Can you work these out from the model? Positions are in its coordinate system, mm. Give positions to 0.01 mm unless a question says otherwise; leave off trailing zeros. Order: outer loops, then holes, each group sorted by start corner. A loop starts at its lowest first (then second) coordinate and runs counter-clockwise, first axis right, second up. Notation, with made-up numbers: (38.25, 48) - (57.25, 48) arc R13 ccw to (57.25, 67) - close; hole circle Ø9 at (78.25, 9.25). An arc over 180 degrees is marked (long way). One line per question, with ' | ' between items.
```python
from build123d import *

# Parameters (mm, degrees)
BOSS_EXTRUDE1_DEPTH      = 3.175
BOSS_EXTRUDE1_DEPTH_BACK = 3.175
CUT_EXTRUDE3_DEPTH       = 206.528461822
CUT_EXTRUDE5_DEPTH       = 206.528461822
CUT_EXTRUDE6_DEPTH       = 6.35
SKETCH8_W                = 3.175
SKETCH8_H                = 3.175
CUT_EXTRUDE7_DEPTH       = 6.35


with BuildPart() as part:
    # Sketch1 → Boss-Extrude1 (new, two sides: drawn at the far end of the back side and taken through both)
    with BuildSketch(Plane.XY.offset(-BOSS_EXTRUDE1_DEPTH_BACK)):
        with BuildLine():
            Line((-95.480291898, -80.706386575), (-95.480291898, -131.085242165))
            Line((-95.480291898, -131.085242165), (-95.480291898, -132.672742165))
            Line((-95.480291898, -132.672742165), (-120.480291898, -132.672742165))
            Line((-120.480291898, -132.672742165), (-120.480291898, -131.085242165))
            Line((-120.480291898, -131.085242165), (-120.480291898, -64.018285781))
            ThreePointArc((-120.480291898, -64.018285781), (-115.755703828, -49.392703021), (-103.367678212, -40.295108567))
            Line((-103.367678212, -40.295108567), (119.519708102, 33.809591006))
            Line((119.519708102, 33.809591006), (119.519708102, 8.809591006))
            Line((119.519708102, 8.809591006), (-78.367678212, -56.983209361))
            ThreePointArc((-78.367678212, -56.983209361), (-90.755703828, -66.080803815), (-95.480291898, -80.706386575))
        make_face()
    extrude(amount=BOSS_EXTRUDE1_DEPTH + BOSS_EXTRUDE1_DEPTH_BACK)

    # Sketch2 → Cut-Extrude3 (cut, through all)
    with BuildSketch(Plane.XZ.offset(132.672742165)):
        Polygon((-120.480291898, 0), (-120.480291898, 3.175), (-118.647204793, 3.175), align=None)
    cut_extrude3 = extrude(amount=-CUT_EXTRUDE3_DEPTH, mode=Mode.SUBTRACT)

    # Mirror3: Cut-Extrude3 across plane
    add(cut_extrude3.mirror(Plane.XY), mode=Mode.SUBTRACT)

    # Sketch3 → Cut-Extrude5 (cut, through all)
    with BuildSketch(Plane.XZ.offset(132.672742165)):
        Polygon((119.519708102, 3.175), (114.020446788, 3.175), (119.519708102, 0), align=None)
    cut_extrude5 = extrude(amount=-CUT_EXTRUDE5_DEPTH, mode=Mode.SUBTRACT)

    # Mirror4: Cut-Extrude5 across plane
    add(cut_extrude5.mirror(Plane.XY), mode=Mode.SUBTRACT)

    # Sketch6 → Cut-Extrude6 (cut)
    with BuildSketch(Plane.XY.offset(3.175)):
        Polygon((33.546459297, -19.774448133), (38.29109474, -18.19697087), (35.769730347, -16.267373348), (31.025094904, -17.844850611), align=None)
    extrude(amount=-CUT_EXTRUDE6_DEPTH, mode=Mode.SUBTRACT)

    # Sketch8 → Cut-Extrude7 (cut)
    with BuildSketch(Plane.XY.offset(3.175)):
        with Locations((-97.067791898, -84.378992165)):
            Rectangle(SKETCH8_W, SKETCH8_H)
    extrude(amount=-CUT_EXTRUDE7_DEPTH, mode=Mode.SUBTRACT)


solid = part.part
```
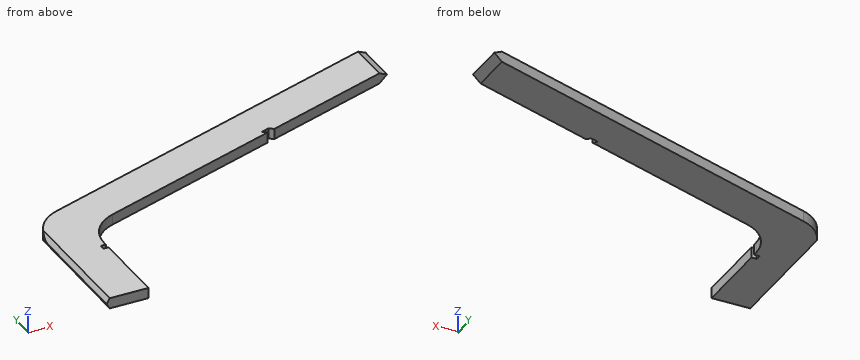
(1) If I drill on line 1 (X direction, y = -73.5, z = -1.25); line 2 (Y direction, x = -3, z = -1.25); line 3 (X direction, y = -60, z = -1.25), over which ranges is the centre line in solid material (lowest first)?
Answer below:
line 1: -119.76 to -94.42 | line 2: -31.93 to -6.93 | line 3: -119.76 to -84.49
(2) Imagine slicing it at A-A (z = -1.75). List the corners of the cut face in (x, y) for me, and give its area (3 significant figures).
Answer below:
outline: (-119.47, -132.67) - (-95.48, -132.67) - (-95.48, -85.97) - (-98.66, -85.97) - (-98.66, -82.79) - (-95.48, -82.79) - (-95.48, -80.71) arc R25 cw to (-78.37, -56.98) - (33.55, -19.77) - (31.03, -17.84) - (35.77, -16.27) - (38.29, -18.2) - (116.49, 7.8) - (116.49, 32.8) - (-103.37, -40.3) arc R25 ccw to (-119.47, -56.98) - close | area: 7,470 mm^2
(3) Will these pins go through, and if not, where does the flat tip stop? pin 1 (1.6 mm diameter, centred on y = -84, z = 1.5, fed in from +X); pin 2 (1.7 mm diameter, centred on y = -82, z = -0.5, fed in from +X); pin 3 (2 mm diameter, centred on x = 81.5, z = 1.5, fed in from +Y).
Answer below:
pin 1: x = -98.66 | pin 2: x = -95.48 | pin 3: y = 21.5
(4) Imagine slicing it at D-D (y = 16). List the corners of the cut face in (x, z) for me (3 decimals), and give its area (3 significant figures).
Answer below:
outline: (65.953, -3.175) - (114.02, -3.175) - (119.52, 0) - (114.02, 3.175) - (65.953, 3.175) - close | area: 323 mm^2
(5) Imagine slicing it at C-C (x = 7.5). List the corners of the cut face in (y, z) for me (3 decimals), and give its area (3 significant figures).
Answer below:
outline: (-28.434, -3.175) - (-3.434, -3.175) - (-3.434, 3.175) - (-28.434, 3.175) - close | area: 159 mm^2
(6) Imagine slicing it at B-B (y = -112). List the corners of the cut face in (x, z) for me (3 decimals).
Answer below:
outline: (-120.48, 0) - (-118.647, -3.175) - (-95.48, -3.175) - (-95.48, 3.175) - (-118.647, 3.175) - close
